Source: three-view drawing plus pictorial views. Frame: mm from the lowest corner of the part. A direction names the side the tool comes from. Coordinates: 2 decimals unless noted, no trailing zeros. Loops run counter-clockwise (first coordinate to the right, second up) from the corner with the lowest first, then second, coordinate; pieces in that order, holes last. Notation, with made-up numbers: (28.5, -38) - (87.5, -38) arc R12 ccw to (87.5, -17) - close; hole circle Ø2 at (-35.5, 37). An arc over 180 degrees is marked (long way). Return JSON: item names as keys, results as strings.
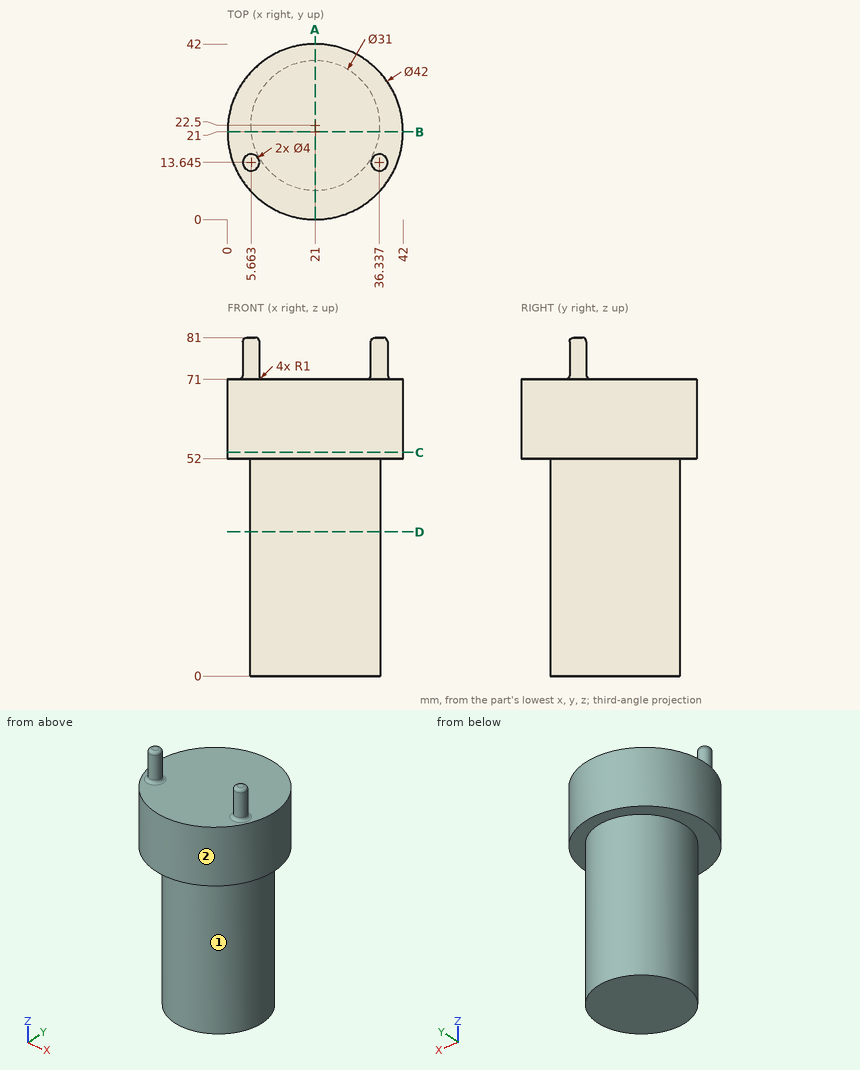
Item 1: Section query C-C, the plane z = 53.5. Return loops of the section in (x, y).
Worked out:
{"outline": "circle Ø42 at (21, 21)"}
Item 2: Section query B-B, the plane y = 21. Return loops of the section in (x, z), and give its area (3 significant figures).
Worked out:
{"outline": "(0, 52) - (5.57, 52) - (5.57, 0) - (36.43, 0) - (36.43, 52) - (42, 52) - (42, 71) - (0, 71) - close", "area": "2,400 mm^2"}
Item 3: Reachability of the marked faces 1 and 2 from +Z, -Z, +X, -X, +Y, -Y: full face, straight path, thin tool, end or side. Return the list, or none.
Worked out:
{"face 1": "-Z", "face 2": "+Z, -Z"}
Item 4: Section query A-A, the plane x = 21. Return loops of the section in (y, z).
Worked out:
{"outline": "(0, 52) - (7, 52) - (7, 0) - (38, 0) - (38, 52) - (42, 52) - (42, 71) - (0, 71) - close"}
Item 5: Section query D-D, the plane z = 34.5. Return loops of the section in (x, y), and give its area (3 significant figures).
Worked out:
{"outline": "circle Ø31 at (21, 22.5)", "area": "755 mm^2"}
Item 6: Ray query, probe 1 along Z at (x, y) = (37, 8); probe 2 along Z at (x, y) = (8, 27.5); probe 3 along X at (y, z) = (23, 34). Return the intervals inside material, ascending. Write a range as from..to.
Worked out:
{"probe 1": "52..71", "probe 2": "0..71", "probe 3": "5.51..36.49"}
Item 7: First-contact query: pin 1 Ø10 at (x, z) = (15, 19) entering from +Y; pin 2 Ø1.5 at (x, y) = (7.5, 8) entering from -Z; pin 3 Ø6 at (y, z) = (22.5, 26) entering from -X. Flat tips, straight axial feed; report the tip coordinate or a pass-through.
Worked out:
{"pin 1": "y = 37.97", "pin 2": "z = 52", "pin 3": "x = 5.5"}
